The listing builds one solid part. Answer for the finished solid, in the listing's coordinates (mm). Round coordinates to 2 decimals unless told otherwise and drop trailing zeros. Write each loop counter-clockwise with the first axis right and the second up, starting at its lowest first coordinate (ties: lowest second). Pieces come first, ordered by that corner, then holes. Notation, with made-up numbers: M 89.5,75 L 106.5,75 A24 cw 106.5,95 Z; hole C 73.25,50.5 d11. An arc over 180 degrees is marked long. One line per item, written item: value. Start each with the question number.
(1) Consider probe 1 along X at (y, z) = (0, 10); probe 2 along Y at (x, z) = (0, 9.75). Determine where each line is inside the solid, lowest interval first.
(2) Section B-B (x = 0) is taken. Determine the outline of the cut face in (y, z), plus the area to 3 significant figures.
(3) Section A-A (y = 0) is taken. Determine the outline of the cut face in (x, z), plus the area to 3 significant figures.
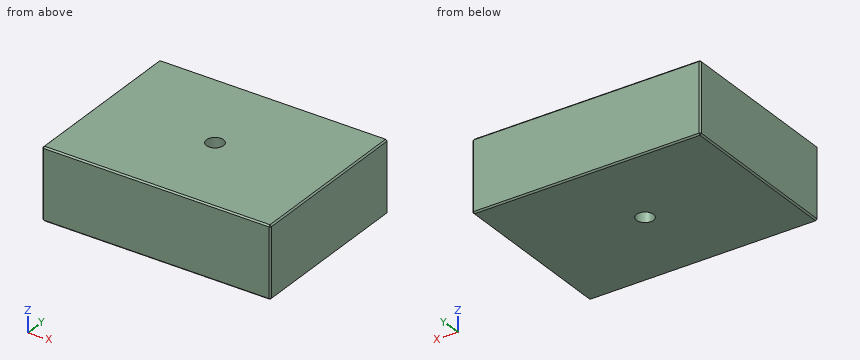
```python
from build123d import *

# Parameters (mm, degrees)
SKETCH_W     = 80
SKETCH_H     = 60
PAD_DEPTH    = 25
SKETCH001_R  = 3
POCKET_DEPTH = 25.001
CHAMFER_SIZE = 0.5


with BuildPart() as part:
    # Sketch → Pad (new body)
    with BuildSketch(Plane.XY):
        Rectangle(SKETCH_W, SKETCH_H)
    extrude(amount=PAD_DEPTH)

    # Sketch001 → Pocket (cut, through all)
    with BuildSketch(Plane.XY):
        Circle(SKETCH001_R)
    extrude(amount=POCKET_DEPTH, mode=Mode.SUBTRACT)

    # Chamfer
    chamfer_edges = [part.edges().sort_by_distance(p)[0] for p in [
        (-40, -30, 12.5),
        (40, -30, 12.5),
        (0, -30, 0),
        (0, -30, 25),
        (40, 30, 12.5),
        (40, 0, 0),
        (40, 0, 25),
        (-40, 30, 12.5),
        (-40, 0, 0),
        (-40, 0, 25),
        (0, 30, 0),
        (0, 30, 25),
    ]]
    chamfer(chamfer_edges, length=CHAMFER_SIZE)


solid = part.part
```
Recorded:
1. probe 1: x = -40 to -3, 3 to 40
1. probe 2: y = -30 to -3, 3 to 30
2. outline: M -30,0.5 L -29.5,0 L -3,0 L -3,25 L -29.5,25 L -30,24.5 Z; M 3,0 L 29.5,0 L 30,0.5 L 30,24.5 L 29.5,25 L 3,25 Z
2. area: 1,350 mm2
3. outline: M -40,0.5 L -39.5,0 L -3,0 L -3,25 L -39.5,25 L -40,24.5 Z; M 3,0 L 39.5,0 L 40,0.5 L 40,24.5 L 39.5,25 L 3,25 Z
3. area: 1,850 mm2
